Can you work these out from the model? Positions are in its coordinate system, mm. Face numbers are marked on the shaded views. A direction names the side the tool comes from. Round coordinates to 2 decimals unless told otherwise and drop trailing zeros. Order: outer loops, then holes, each group sorted by start corner. A loop starts at its lowest first (then second) coordinate and runs counter-clockwise, first axis right, second up.
Q1. If we section it at C-C (z = 1): Please give me the cut outline in (x, y), plus the area to 3 significant figures.
Q2. We'd pull the mould along Z, two halves only. Please class the marked faces 5, 6 and 7: pulls with the +Z half, pulls with the -Z half, needs draft (parallel to the pull), parting line crosses it, or undercut.
Q3. If we section it at B-B (x = 0): Please give me the cut outline in (y, z), plus the area to 3 significant figures.
Q4. If we section it at D-D (x = 21): Count the separate pieces of the cut face and the enclosed holes in it, plus the area to 3 significant figures.
Q5. If we section it at A-A (y = -4): Please give me the cut outline in (x, z).
Q6. If I drill on line 1 (Z direction, x = 0, y = -5.25); line 2 (Y direction, x = -21, z = -12.75); line 3 (X direction, y = -6, z = -5.75), over which ranges is the centre line in solid material (lowest first)?
Q7. For the marked faces 1, 2, 3 and 4, which set-ups out of +Z, -Z, +X, -X, +Y, -Y let a thin tool reach every point of the face, with its end or its side?
Q8. Will these pins go through, and if not, where does the flat tip stop? P1, Ø1.5, axis at x = 8, y = -1.5, coming from the -Z side; P2, Ø7.5, axis at x = 17, z = 1.5, coming from the +Y side; P3, Ø6.5, axis at x = 2, y = -4, coming from the +Z side; P4, Ø9.5, axis at x = 20, y = 3, coming from the +Z side.
from build123d import *

# Parameters (mm, degrees)
SKETCH002_R     = 2
SKETCH002_R_2   = 6.5
SKETCH002_R_3   = 3
PAD_DEPTH       = 8
SKETCH003_R     = 7.7
POCKET_DEPTH    = 2
SKETCH004_R     = 3
POCKET001_DEPTH = 31
SKETCH005_R     = 2
PAD001_DEPTH    = 2
SKETCH007_R     = 3
POCKET002_DEPTH = 11


with BuildPart() as part:
    # Sketch002 → Pad (new body)
    with BuildSketch(Plane.XZ):
        with BuildLine():
            Line((-6.339749, 5.000001), (6.339746, 5.000001))
            ThreePointArc((25.000002, 0), (17.588192, 9.659262), (6.339746, 5.000001))
            Line((25.000002, -14.499996), (25.000002, 0))
            Line((15.000002, -14.499996), (25.000002, -14.499996))
            Line((15.000002, -9.999996), (15.000002, -14.499996))
            ThreePointArc((6.339751, -5.000001), (10.000004, -8.660251), (15.000002, -9.999996))
            Line((-6.339746, -5.000001), (6.339751, -5.000001))
            ThreePointArc((-15, -10), (-10, -8.660255), (-6.339746, -5.000001))
            Line((-15, -10), (-15, -14.499996))
            Line((-25, -14.499996), (-15, -14.499996))
            Line((-25, 0), (-25, -14.499996))
            ThreePointArc((-6.339749, 5.000001), (-17.588192, 9.659257), (-25, 0))
        make_face()
        with Locations((-15, 0)):
            Circle(SKETCH002_R, mode=Mode.SUBTRACT)
        with Locations((15.000002, 4e-06)):
            Circle(SKETCH002_R_2, mode=Mode.SUBTRACT)
        Circle(SKETCH002_R_3, mode=Mode.SUBTRACT)
    extrude(amount=PAD_DEPTH)

    # Sketch003 (on Face16 of Pad) → Pocket (cut)
    with BuildSketch(Plane(origin=(0, 0, 0), x_dir=(1, 0, 0), z_dir=(0, 1, 0))):
        with Locations((15.000002, -4e-06)):
            Circle(SKETCH003_R)
    extrude(amount=-POCKET_DEPTH, mode=Mode.SUBTRACT)

    # Sketch004 → Pocket001 (cut, symmetric)
    with BuildSketch(Plane.YZ):
        with Locations((-4, -10)):
            Circle(SKETCH004_R)
    extrude(amount=POCKET001_DEPTH, both=True, mode=Mode.SUBTRACT)

    # Sketch005 → Pad001 (join)
    with BuildSketch(Plane.XY.offset(-14.5)):
        with BuildLine():
            Line((-25.000002, 0), (-15.000002, 0))
            Line((-15.000002, 0), (-15.000002, 3.5))
            ThreePointArc((-15.000002, 3.5), (-20.000002, 8.5), (-25.000002, 3.5))
            Line((-25.000002, 0), (-25.000002, 3.5))
        make_face()
        with Locations((-20.000002, 3.5)):
            Circle(SKETCH005_R, mode=Mode.SUBTRACT)
        with BuildLine():
            Line((15.000002, 0), (25.000002, 0))
            Line((25.000002, 0), (25.000002, 3.5))
            ThreePointArc((25.000002, 3.5), (20.000002, 8.5), (15.000002, 3.5))
            Line((15.000002, 0), (15.000002, 3.5))
        make_face()
        with Locations((20.000002, 3.5)):
            Circle(SKETCH005_R, mode=Mode.SUBTRACT)
    extrude(amount=PAD001_DEPTH)

    # Sketch007 → Pocket002 (cut)
    with BuildSketch(Plane.XZ.offset(2)):
        with Locations((-15, 0)):
            Circle(SKETCH007_R)
    extrude(amount=POCKET002_DEPTH, mode=Mode.SUBTRACT)


solid = part.part
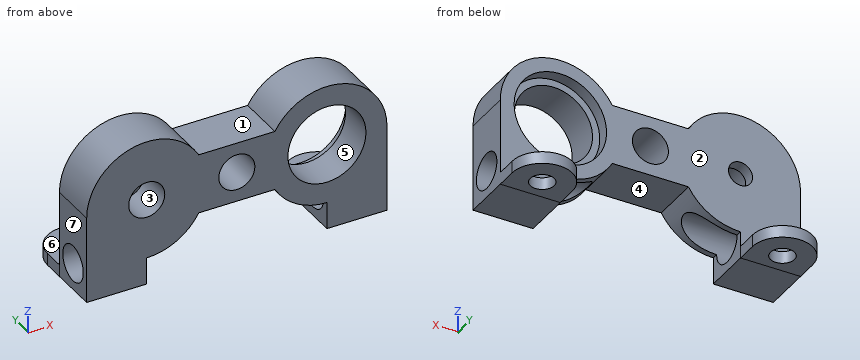
Solution:
1. outline: (-24.95, -8) - (-17.83, -8) - (-17.83, -2) - (-16.73, -2) - (-16.73, 0) - (-24.95, 0) - close; (-13.27, -2) - (-12.17, -2) - (-12.17, -8) - (-2.83, -8) - (-2.83, 0) - (-13.27, 0) - close; (2.83, -8) - (8.58, -8) - (8.58, -2) - (7.37, -2) - (7.37, 0) - (2.83, 0) - close; (21.42, -8) - (24.95, -8) - (24.95, 0) - (22.63, 0) - (22.63, -2) - (21.42, -2) - close
1. area: 205 mm2
2. face 5: undercut
2. face 6: pulls with the +Z half
2. face 7: needs draft
3. outline: (-8, -5) - (0, -5) - (0, -3) - (-8, -3) - close; (-8, 3) - (0, 3) - (0, 5) - (-8, 5) - close
3. area: 32.0 mm2
4. separate pieces: 3
4. enclosed holes: 1
4. area: 112 mm2
5. outline: (-25, -14.5) - (-15, -14.5) - (-15, -13) - (-25, -13) - close; (-25, -7) - (-7.86, -7) arc R10 ccw to (-6.34, -5) - (6.34, -5) arc R10 ccw to (7.86, -7) - (25, -7) - (25, 0) arc R10 ccw to (6.34, 5) - (-6.34, 5) arc R10 ccw to (-25, 0) - close; (15, -14.5) - (25, -14.5) - (25, -13) - (15, -13) - close; hole circle Ø6 at (-15, 0); hole circle Ø6 at (0, 0); hole circle Ø13 at (15, 0)
6. line 1: z = -5 to -3, 3 to 5
6. line 2: y = -8 to -5.2, -2.8 to 1.77, 5.23 to 8.4
6. line 3: x = -25 to -6.82, 6.82 to 11.97, 18.03 to 25
7. face 1: +Z, +Y, -Y
7. face 2: +Z, +X, -X, +Y
7. face 3: -Y
7. face 4: -Z, +Y, -Y
8. P1: stops at z = -7.81
8. P2: passes through
8. P3: stops at z = 5
8. P4: stops at z = 9.91
